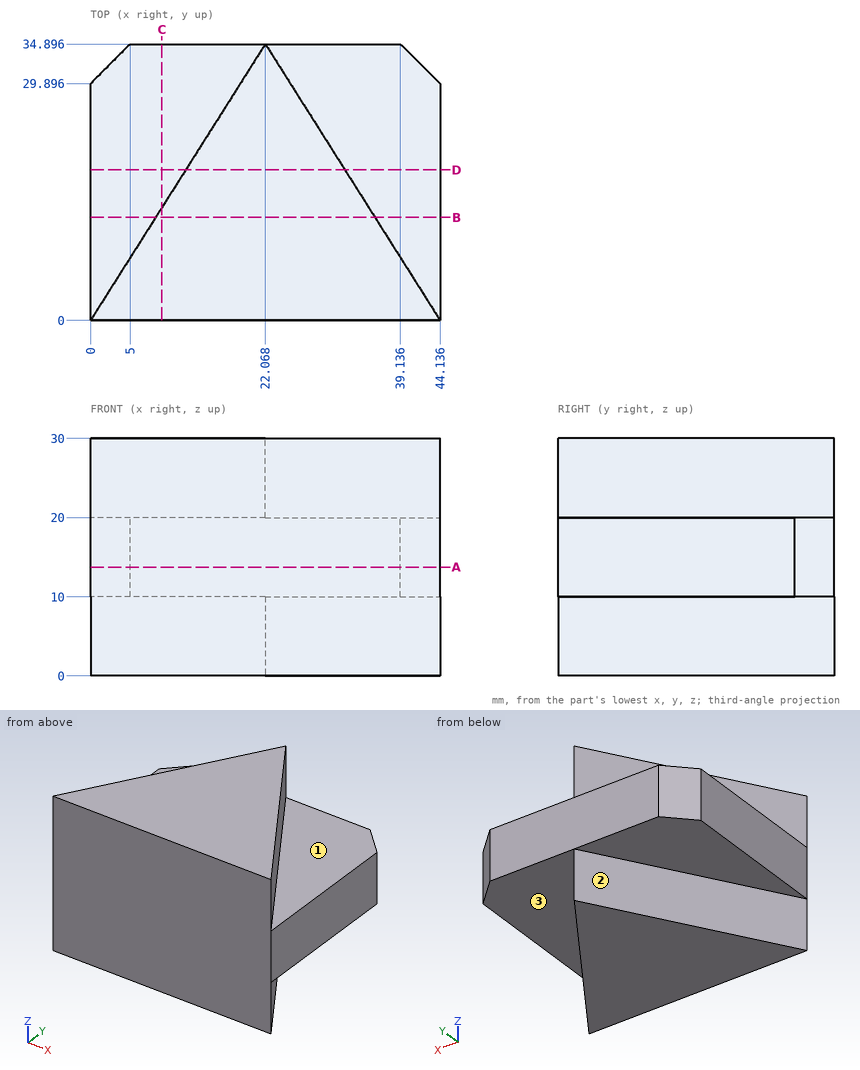
Geometry: see drawing. Coordinates: mm, zero at the bounding-box minimum. A direction names the side the tool comes from. Give positions to 0.01 mm unless a question says otherwise; leave off trailing zeros. Order: outer loops, then holes, each group sorted by start corner. A loop starts at its lowest first (then second) coordinate and runs counter-clockwise, first axis right, second up. Notation, with made-up numbers: M 70.5,66.5 L 109.5,66.5 A23 cw 109.5,74.5 Z; hole C 65,-18.5 d4. An arc over 180 degrees is marked long. Answer as a JSON object with one key per item and string values.
1. First-contact query: P1, Ø1, axis at x = 35.5, z = 21, coming from the +Y side (1 decimal). Flat tip, straight axial feed; report the tip coordinate or a pass-through.
Result sheet:
{"P1": "y = 14.4"}
2. Cut plane C-C, the plane x = 9. Output: boundary loops of the cut face in (y, z).
Result sheet:
{"outline": "M 0,0 L 14.23,0 L 14.23,10 L 34.9,10 L 34.9,20 L 14.23,20 L 14.23,30 L 0,30 Z"}
3. Cut plane D-D, the plane y = 19. Output: boundary loops of the cut face in (x, z) (1 decimal).
Result sheet:
{"outline": "M 0,10 L 12,10 L 12,0 L 32.1,0 L 32.1,10 L 44.1,10 L 44.1,20 L 32.1,20 L 32.1,30 L 12,30 L 12,20 L 0,20 Z"}
4. Cut plane B-B, the plane y = 13. Output: boundary loops of the cut face in (x, z) (1 decimal).
Result sheet:
{"outline": "M 0,10 L 8.2,10 L 8.2,0 L 35.9,0 L 35.9,10 L 44.1,10 L 44.1,20 L 35.9,20 L 35.9,30 L 8.2,30 L 8.2,20 L 0,20 Z"}
5. Ray query, line 1 (Z direction, x = 40.5, y = 16); line 2 (X direction, y = 16, z = 4.25); line 3 (X direction, y = 30, z = 22.5) (1 decimal). Return the intervals inside material, ascending. Write a range as [from, to].
Result sheet:
{"line 1": "[10, 20]", "line 2": "[10.12, 34.02]", "line 3": "[19, 25.2]"}
6. Cut plane A-A, the plane z = 13.75. Output: boundary loops of the cut face in (x, y).
Result sheet:
{"outline": "M 0,0 L 44.14,0 L 44.14,29.9 L 39.14,34.9 L 5,34.9 L 0,29.9 Z"}
7. Reachability of the marked faces 1, 2 and 3 from +Z, -Z, +X, -X, +Y, -Y: full face, straight path, thin tool, end or side. Return the list, or none.
Result sheet:
{"face 1": "+Z, +X, +Y", "face 2": "-Z, -X, +Y", "face 3": "-Z, +X, +Y"}
